Could you check a few things on this model? Use its own coordinates, in mm. A direction names the side the tool comes from. Round coordinates to 2 decimals unless told otherwise and drop trailing zeros. Loops run counter-clockwise (first coordinate to the right, second up) from the corner with the lowest first, then second, coordinate; pieces in that order, holes last. Notation, with made-up numbers: (61, 13.25) - (86, 13.25) arc R26 cw to (86, 32.25) - close; hole circle Ø8 at (1, 54). An arc over 180 degrees is marked (long way). Answer as CSV lines item,"result". Start each with the question number.
1) Which directions (+Z, -Z, +X, -X, +Y, -Y) give clear straight access to the entire face, cutting with the end or side of a thin tool? Please do faces 1 (the face through (-6, 0, 9)), 2 (the face through (0, 2.8, 6.7)), 3 (the face through (-32.97, -8.18, 8.63)), 4 (the face through (75.35, 7.276, 10.102)).
2) I'm going to push flat-ended pins straight in: pin 1 Ø2.5 at (y, z) = (8.75, 8.75) entering from +X; pin 2 Ø5 at (y, z) = (-5, 12.5) entering from +X (3 decimals); pin 3 Ø6 at (y, z) = (-10, 2.5) entering from -X. Where does each tip first touch, or does it pass through?
3) Suppose I cut it at A-A, the plane x = 54.5. Write out the boundary of the cut face in (y, z).
4) We'd pull the mould along Y, two halves only. Please class faces 5 (the face through (-26, -25, 9)), 6 (the face through (100, 9, 11)), 7 (the face through (50, 9, 9)): pulls with the +Y half, pulls with the -Y half, needs draft (parallel to the pull), parting line crosses it, or undercut.
5) Suppose I cut it at B-B, the plane z = 8.75. Write out the boundary of the cut face in (x, y).
6) Suppose I cut it at D-D, the plane y = -19. Write out the boundary of the cut face in (x, z), then the cut area to 3 significant figures.
7) Suppose I cut it at C-C, the plane y = -11. Write out the boundary of the cut face in (x, z), then the cut area to 3 significant figures.
8) Please list where these lines run through material, in increasing order: line 1 along Y through (x, z) = (84.25, 16); line 2 along X through (y, z) = (8.75, 2.5); line 3 along Z through (x, y) = (73, 8.75).
```python
from build123d import *

# Parameters (mm, degrees)
BOSS_EXTRUDE4_START = 5
SKETCH2_W           = 17.5
SKETCH2_H           = 17.5
BOSS_EXTRUDE4_DEPTH = 95
SKETCH3_R           = 2
CUT_EXTRUDE1_DEPTH  = 50
SKETCH4_R           = 1
CUT_EXTRUDE2_DEPTH  = 50
SKETCH6_R           = 6
BOSS_EXTRUDE6_DEPTH = 5
BOSS_EXTRUDE8_DEPTH = 17.5


with BuildPart() as part:
    # Sketch2 → Boss-Extrude4 (new body)
    with BuildSketch(Plane(origin=(0, 0, 0), x_dir=(0, 0, -1), z_dir=(1, 0, 0)).offset(BOSS_EXTRUDE4_START)):
        with Locations((-8.75, 8.75)):
            Rectangle(SKETCH2_W, SKETCH2_H)
    extrude(amount=BOSS_EXTRUDE4_DEPTH)

    # Sketch3 → Cut-Extrude1 (cut)
    with BuildSketch(Plane(origin=(100, 0, 0), x_dir=(0, 0, -1), z_dir=(1, 0, 0))):
        with Locations(Location((-8.75, 8.75, 0), (0, 0, 90))):
            Circle(SKETCH3_R)
    extrude(amount=-CUT_EXTRUDE1_DEPTH, mode=Mode.SUBTRACT)

    # Sketch4 → Cut-Extrude2 (cut)
    with BuildSketch(Plane(origin=(0, 0, 0), x_dir=(-1, 0, 0), z_dir=(0, 0, -1))):
        with Locations((-84.25, 8.75)):
            Circle(SKETCH4_R)
    extrude(amount=-CUT_EXTRUDE2_DEPTH, mode=Mode.SUBTRACT)

    # Sketch6 → Boss-Extrude6 (add)
    with BuildSketch(Plane.ZY.offset(-5)):
        with Locations((8.75, 8.75)):
            Circle(SKETCH6_R)
    extrude(amount=BOSS_EXTRUDE6_DEPTH)

    # Sketch1 → Boss-Extrude8 (add)
    with BuildSketch(Plane.XY):
        with BuildLine():
            Line((0, 17.5), (-25.582464074, 17.5))
            ThreePointArc((-25.582464074, 17.5), (-33.242908505, 13.927876097), (-35.430541604, 5.763518223))
            Line((-35.430541604, 5.763518223), (-30.443227685, -22.520944533))
            ThreePointArc((-30.443227685, -22.520944533), (-29.417167255, -24.298133329), (-27.488804426, -25))
            Line((-27.488804426, -25), (-24.280949674, -25))
            ThreePointArc((-24.280949674, -25), (-22.468303976, -24.390463464), (-21.392240798, -22.809543714))
            Line((-21.392240798, -22.809543714), (-15.818483363, -2.920608381))
            ThreePointArc((-15.818483363, -2.920608381), (-14.383732459, -0.812715382), (-11.966871527, 0))
            Line((-11.966871527, 0), (0, 0))
            Line((0, 0), (0, 17.5))
        make_face()
    extrude(amount=BOSS_EXTRUDE8_DEPTH)


solid = part.part
```
Filled sheet:
1,face 1,"+Z, -Z, +X, -Y"
1,face 2,"none"
1,face 3,"+Z, -Z, -X, -Y"
1,face 4,"+X"
2,pin 1,"x = 50"
2,pin 2,"x = -15.675"
2,pin 3,"x = -33.18"
3,outline,"(0, 0) - (17.5, 0) - (17.5, 17.5) - (0, 17.5) - close; hole circle Ø4 at (8.75, 8.75)"
4,face 5,"pulls with the -Y half"
4,face 6,"needs draft"
4,face 7,"undercut"
5,outline,"(-35.43, 5.76) - (-30.44, -22.52) arc R3 ccw to (-27.49, -25) - (-24.28, -25) arc R3 ccw to (-21.39, -22.81) - (-15.82, -2.92) arc R4 cw to (-11.97, 0) - (0, 0) - (0, 2.75) - (5, 2.75) - (5, 0) - (100, 0) - (100, 6.75) - (50, 6.75) - (50, 10.75) - (100, 10.75) - (100, 17.5) - (5, 17.5) - (5, 14.75) - (0, 14.75) - (0, 17.5) - (-25.58, 17.5) arc R10 ccw to start"
6,outline,"(-31.06, 0) - (-20.32, 0) - (-20.32, 17.5) - (-31.06, 17.5) - close"
6,area,"188 mm²"
7,outline,"(-32.47, 0) - (-18.08, 0) - (-18.08, 17.5) - (-32.47, 17.5) - close"
7,area,"252 mm²"
8,line 1,"0 to 7.75, 9.75 to 17.5"
8,line 2,"-35.5 to 0, 5 to 83.25, 85.25 to 100"
8,line 3,"0 to 6.75, 10.75 to 17.5"
